Work out the finished part from the listing and answer in its coordinate system (mm). A direction names the side the tool comes from. Give positions to 0.01 mm unless a question says otherwise; leave off trailing zeros. Loops run counter-clockwise (first coordinate to the right, second up) from the corner with the lowest first, then second, coordinate; pieces in that order, holes last. Notation, with made-up numbers: (61, -8) - (82, -8) arc R24 ccw to (82, 28) - close; hole circle Ø3 at (31.25, 62). An arc over 180 degrees is marked (long way). One line per item, written item: value.
from build123d import *

# Parameters (mm, degrees)
SKETCH1_R           = 1.25
BOSS_EXTRUDE1_DEPTH = 1
BOSS_EXTRUDE2_DEPTH = 8
CUT_EXTRUDE1_DEPTH  = 3.2
SKETCH4_R           = 1.6
BOSS_EXTRUDE3_DEPTH = 3
CHAMFER1_SIZE       = 1.55
CHAMFER2_SIZE       = 1.55
CHAMFER3_SIZE       = 1.55
SKETCH5_W           = 8.5
SKETCH5_H           = 12.5
CUT_EXTRUDE2_DEPTH  = 3
CHAMFER4_SIZE       = 3
CHAMFER5_SIZE       = 1.45
SKETCH6_W           = 8.5
SKETCH6_H           = 3.2
CUT_EXTRUDE3_DEPTH  = 69.023892861


# Some blends are built 0.0001 mm under size
with BuildPart() as part:
    # Sketch1 → Boss-Extrude1 (new body)
    with BuildSketch(Plane.XY):
        Polygon((0, 0), (0, 4.5), (8.5, 4.5), (8.5, 12), (17, 12), (17, 0), (17, -12.5), (8.5, -12.5), (8.5, 0), align=None)
        with Locations((2.15, 2.35)):
            Circle(SKETCH1_R, mode=Mode.SUBTRACT)
    extrude(amount=BOSS_EXTRUDE1_DEPTH)

    # Sketch2 → Boss-Extrude2 (add)
    with BuildSketch(Plane.XY.offset(1)):
        Polygon((5.15, 4.5), (5.15, 0), (8.5, 0), (8.5, -12.5), (17, -12.5), (17, 12), (8.5, 12), (8.5, 4.5), align=None)
    extrude(amount=BOSS_EXTRUDE2_DEPTH)

    # Sketch3 → Cut-Extrude1 (cut)
    with BuildSketch(Plane.XY.offset(9)):
        Polygon((8.5, 10), (17, 10), (17, -10.5), (8.5, -10.5), (5.15, -10.5), (5.15, 4.5), (8.5, 4.5), align=None)
    extrude(amount=-CUT_EXTRUDE1_DEPTH, mode=Mode.SUBTRACT)

    # Sketch4 → Boss-Extrude3 (add)
    with BuildSketch(Plane(origin=(17, 0, 0), x_dir=(0, 0, -1), z_dir=(1, 0, 0))):
        Polygon((-5.8, 0), (61, 0), (61, 4.5), (61, 7.5), (36, 7.5), (36, 4.5), (-5.8, 4.5), align=None)
        with Locations(Location((57, 5, 0), (0, 0, 90))):
            Circle(SKETCH4_R, mode=Mode.SUBTRACT)
        with Locations(Location((45, 5, 0), (0, 0, 90))):
            Circle(SKETCH4_R, mode=Mode.SUBTRACT)
    extrude(amount=BOSS_EXTRUDE3_DEPTH)

    # Chamfer1
    # the kernel refuses this chamfer: 1.55 mm, written as the material it takes off along each edge
    with BuildSketch(Plane(origin=(20, 5, -57), x_dir=(0, 1, 0), z_dir=(0, 0, -1))) as chamfer1_piece_1:
        Polygon((1.6, -CHAMFER1_SIZE), (1.6 + CHAMFER1_SIZE, 0), (1.6, 0), align=None)
    revolve(axis=Axis((20, 5, -57), (1, 0, 0)), mode=Mode.SUBTRACT)
    with BuildSketch(Plane(origin=(20, 5, -45), x_dir=(0, 1, 0), z_dir=(0, 0, -1))) as chamfer1_piece_2:
        Polygon((1.6, -CHAMFER1_SIZE), (1.6 + CHAMFER1_SIZE, 0), (1.6, 0), align=None)
    revolve(axis=Axis((20, 5, -45), (1, 0, 0)), mode=Mode.SUBTRACT)

    # Chamfer2
    # the kernel refuses this chamfer: 1.55 mm, written as the material it takes off along each edge
    with BuildSketch(Plane(origin=(20, 7.5, -59.069731842), x_dir=(0.027495876610587087, -0.9996219169112966, 0), z_dir=(0, 0, 1))) as chamfer2_piece_1:
        Polygon((CHAMFER2_SIZE * 0.999621916911, -CHAMFER2_SIZE * 0.0274958766106), (-CHAMFER2_SIZE * 0.0274958766106, -CHAMFER2_SIZE * 0.999621916911), (0, 0), align=None)
    extrude(amount=16.139463683, mode=Mode.SUBTRACT)
    with BuildSketch(Plane(origin=(20, 7.5, -47.069731842), x_dir=(0.027495876610587087, -0.9996219169112966, 0), z_dir=(0, 0, 1))) as chamfer2_piece_2:
        Polygon((CHAMFER2_SIZE * 0.999621916911, -CHAMFER2_SIZE * 0.0274958766106), (-CHAMFER2_SIZE * 0.0274958766106, -CHAMFER2_SIZE * 0.999621916911), (0, 0), align=None)
    extrude(amount=15.055840473, mode=Mode.SUBTRACT)
    with BuildSketch(Plane(origin=(20.986108631, 12, 9), x_dir=(0, 0.02749587661058596, -0.9996219169112966), z_dir=(-1, 0, 0))) as chamfer2_piece_3:
        Polygon((CHAMFER2_SIZE * 0.999621916911, CHAMFER2_SIZE * 0.0274958766106), (-CHAMFER2_SIZE * 0.0274958766106, CHAMFER2_SIZE * 0.999621916911), (0, 0), align=None)
    extrude(amount=16.472217263, mode=Mode.SUBTRACT)
    with BuildSketch(Plane(origin=(20, 7.5, -64.986108631), x_dir=(0.027495876610587087, -0.9996219169112966, 0), z_dir=(0, 0, 1))) as chamfer2_piece_4:
        Polygon((CHAMFER2_SIZE * 0.999621916911, -CHAMFER2_SIZE * 0.0274958766106), (-CHAMFER2_SIZE * 0.0274958766106, -CHAMFER2_SIZE * 0.999621916911), (0, 0), align=None)
    extrude(amount=10.055840473, mode=Mode.SUBTRACT)
    with BuildSketch(Plane(origin=(20, 11.486108631, -36), x_dir=(0.027495876610587163, 0, -0.9996219169112966), z_dir=(0, -1, 0))) as chamfer2_piece_5:
        Polygon((CHAMFER2_SIZE * 0.999621916911, -CHAMFER2_SIZE * 0.0274958766106), (-CHAMFER2_SIZE * 0.0274958766106, -CHAMFER2_SIZE * 0.999621916911), (0, 0), align=None)
    extrude(amount=6.986108631, mode=Mode.SUBTRACT)
    with BuildSketch(Plane(origin=(20, 4.5, -36), x_dir=(-0.9996219169112966, 0.027495876610585928, 0), z_dir=(0, 0, 1))) as chamfer2_piece_6:
        Polygon((CHAMFER2_SIZE * 0.999621916911, CHAMFER2_SIZE * 0.0274958766106), (-CHAMFER2_SIZE * 0.0274958766106, CHAMFER2_SIZE * 0.999621916911), (0, 0), align=None)
    extrude(amount=45.786108631, mode=Mode.SUBTRACT)
    with BuildSketch(Plane(origin=(20, 4.5, -39.986108631), x_dir=(-0.9996219169112966, 0.027495876610585928, 0), z_dir=(0, 0, 1))) as chamfer2_piece_7a_section:
        Polygon((CHAMFER2_SIZE * 0.999621916911, CHAMFER2_SIZE * 0.0274958766106), (-CHAMFER2_SIZE * 0.0274958766106, CHAMFER2_SIZE * 0.999621916911), (0, 0), align=None)
    chamfer2_piece_7a = extrude(amount=49.772217263, mode=Mode.PRIVATE)
    chamfer2_piece_7a = split(chamfer2_piece_7a, bisect_by=Plane(origin=(19.488819878, 3.988819878, -36), z_dir=(0, 0, -1)), keep=Keep.TOP, mode=Mode.PRIVATE)
    with BuildSketch(Plane(origin=(20, 11.486108631, -36), x_dir=(0.027495876610587163, 0, -0.9996219169112966), z_dir=(0, -1, 0))) as chamfer2_piece_7b_section:
        Polygon((CHAMFER2_SIZE * 0.999621916911, -CHAMFER2_SIZE * 0.0274958766106), (-CHAMFER2_SIZE * 0.0274958766106, -CHAMFER2_SIZE * 0.999621916911), (0, 0), align=None)
    chamfer2_piece_7b = extrude(amount=10.972217263, mode=Mode.PRIVATE)
    chamfer2_piece_7b = split(chamfer2_piece_7b, bisect_by=Plane(origin=(19.488819878, 4.5, -36.511180122), z_dir=(0, -1, 0)), keep=Keep.TOP, mode=Mode.PRIVATE)
    chamfer2_piece_7 = chamfer2_piece_7a & chamfer2_piece_7b
    add(chamfer2_piece_7, mode=Mode.SUBTRACT)

    # Chamfer3
    chamfer3_edges = [part.edges().sort_by_distance(p)[0] for p in [
        (12.75, -12.5, 9),
        (20, 0, -27.6),
    ]]
    chamfer(chamfer3_edges, length=CHAMFER3_SIZE)

    # Sketch5 → Cut-Extrude2 (cut)
    with BuildSketch(Plane(origin=(0, 0, 0), x_dir=(-1, 0, 0), z_dir=(0, 0, -1))):
        with Locations((-12.75, -6.25)):
            Rectangle(SKETCH5_W, SKETCH5_H)
    extrude(amount=-CUT_EXTRUDE2_DEPTH, mode=Mode.SUBTRACT)

    # Chamfer4
    chamfer4_edges = [part.edges().sort_by_distance(p)[0] for p in [
        (12.75, 0, 3),
        (8.5, 0, 4.4),
    ]]
    chamfer(chamfer4_edges, length=CHAMFER4_SIZE - 0.0001)  # a hair under: the kernel refuses the full size

    # Chamfer5
    chamfer5_edges = [part.edges().sort_by_distance(p)[0] for p in [
        (17, 0, 2.90005),
    ]]
    chamfer(chamfer5_edges, length=CHAMFER5_SIZE - 0.0001)  # a hair under: the kernel refuses the full size
    chamfer5_2_edges = [part.edges().sort_by_distance(p)[0] for p in [
        (18.44995, 0, 5.8),
    ]]
    chamfer(chamfer5_2_edges, length=CHAMFER5_SIZE)

    # Sketch6 → Cut-Extrude3 (cut, through all)
    with BuildSketch(Plane.XZ.offset(-10)):
        with Locations((12.75, 7.4)):
            Rectangle(SKETCH6_W, SKETCH6_H)
    extrude(amount=-CUT_EXTRUDE3_DEPTH, mode=Mode.SUBTRACT)


solid = part.part
1. The mould has two halves that part along X. Classify faces 6 (the flat face through (18, 7.5, -49)), 7 (the conical face through (18.72, 3.13, -56.92)), 8 (the cylindrical face through (1.88, 1.13, 0.49)): released by +X, released by -X, zero draft, split by the parting line, or undercut.
Output:
face 6: zero draft
face 7: released by +X
face 8: undercut
2. For faces 1 (the flat face through (19.21, 3.74, -16.18)), 2 (the flat face through (18, 6, -36)), 3 (the flat face through (6, 4.5, 2)), 4 (the flat face through (17, -8, 5)), 5 (the flat face through (4, 2, 1)), determine the directions among +Z, -Z, +X, -X, +Y, -Y from which every point of the face is accessible in a straight line to the end or side of a thin tool.
Output:
face 1: +Z, +X, +Y
face 2: +Z, +X, -X, +Y
face 3: +Z, -Z, -X, +Y
face 4: +Z, -Z, +X, -Y
face 5: +Z, -X, +Y, -Y
3. Section A-A (z = -57) is taken. Write down the section's boundary in (x, y).
Output:
outline: (17, 0) - (18.45, 0) - (20, 1.55) - (20, 1.85) - (18.45, 3.4) - (17, 3.4) - close; (17, 6.6) - (18.45, 6.6) - (18.9, 7.05) - (18.45, 7.5) - (17, 7.5) - close
4. Find the intervals of material crossed by line 1 along Z through (x, y) = (17.4, 5); line 2 along Y through (x, z) = (2.15, 0.3); line 3 along Z through (x, y) = (16, 3.5), in increasing order.
Output:
line 1: z = -61 to -58.6, -55.4 to -46.6, -43.4 to -36
line 2: y = 0 to 1.1, 3.6 to 4.5
line 3: z = 0 to 5.8
5. Flat-ended cylindrical pins translate along their axes: pin 1 Ø4 at (y, z) = (2, -28.5) entering from -X; pin 2 Ø6 at (x, y) = (12, 3.5) entering from -Z; pin 3 Ø12 at (x, y) = (9.5, 2.5) entering from +Z. Find the tip coordinate at first contact, or state that the pin passes through.
Output:
pin 1: stops at x = 17
pin 2: stops at z = 0
pin 3: stops at z = 5.8
6. Section D-D (y = -7.5) is taken. Write down the section's boundary in (x, z), and give its area (3 significant figures).
Output:
outline: (8.5, 3) - (17, 3) - (17, 5.8) - (8.5, 5.8) - close
area: 23.8 mm²
7. Section B-B (x = 2.15) is taken. Write down the section's boundary in (y, z).
Output:
outline: (0, 0) - (1.1, 0) - (1.1, 1) - (0, 1) - close; (3.6, 0) - (4.5, 0) - (4.5, 1) - (3.6, 1) - close
